Could you check a few things on this model? Use its own coordinates, in mm. A direction names the side the tool comes from. Round coordinates to 2 decimals unless told otherwise and drop trailing zeros. One line per item, written item: value. Start each with the question number.
(1) Thinking about a two-plate mould opening in Z: for faces 3 (the face through (2.849, -18.246, -5.028)), 4 (the face through (-9, -33.139, 3)), 5 (the face through (-2.9, -18.2, -5)), which applies, released by +Z, released by -Z, zero draft, split by the parting line, or undercut?
(2) Which directions (+Z, -Z, +X, -X, +Y, -Y) give clear straight access to the entire face, cutting with the end or side of a thin tool? Please do faces 1 (the face through (1.699, -3.219, -3.267)), 2 (the face through (-2.849, -18.246, 5.028)).
(3) If I drill on L1, parallel to X at y = -30.55, z = 0; L2, parallel to X at y = -12, z = 0; L3, parallel to Z at x = 0, y = -4.25, over which ranges is the centre line in solid material (lowest first)?
(4) I'm going to push flat-ended pins straight in: pin 1 Ø2 at (x, y) = (-2, -8.5) entering from -Z; pin 2 Ø4 at (y, z) = (-24.5, -1.5) entering from -X; pin 3 Ø1 at (x, z) = (-3, -5) entering from -Y; pin 4 Ø1.7 at (x, z) = (2.5, -5.5) entering from -Y. Where does each tip first touch, or does it pass through?
```python
from build123d import *

# Parameters (mm, degrees)
F0_R     = 9.525
F1_DEPTH = 15.24
F3_DEPTH = 8.89
F4_R     = 3.683
F5_DEPTH = 6.351
F8_R     = 2.54
F9_DEPTH = 15.24


# Not quite as in the source:
# - a feature names something its author has since deleted; it is built from what else it names


with BuildPart() as f1:
    # F0 (on Front) → F1 (new body)
    with BuildSketch(Plane.XZ):
        Circle(F0_R)
    extrude(amount=F1_DEPTH)

    # F2 (on face) → F3 (cut)
    with BuildSketch(Plane.XZ.offset(15.24)):
        Polygon((5.7785, -3.3362185305), (5.7785, 3.3362185305), (0, 6.672437061), (-5.7785, 3.3362185305), (-5.7785, -3.3362185305), (0, -6.672437061), align=None)
    extrude(amount=-F3_DEPTH, mode=Mode.SUBTRACT)

    # F4 (on face) → F5 (cut, through all)
    with BuildSketch(Plane.XZ.offset(6.35)):
        Circle(F4_R)
    extrude(amount=-F5_DEPTH, mode=Mode.SUBTRACT)

    # F6 (on Right) → F7 (revolve)
    with BuildSketch(Plane.YZ):
        with BuildLine():
            Line((-33.139064908, -6.672437061), (-33.139064908, -14.292437061))
            add(Edge.make_bspline(
                [(0, -9.4667123631), (-6.0169453004, -12.6291806394), (-11.4998287108, -14.4075187704), (-18.7425000775, -24.446910043), (-30.9530390066, -25.1909209173), (-33.139064908, -14.292437061)],
                knots=[0, 0, 0, 0, 0.3337672016, 0.635034675, 1, 1, 1, 1], degree=3))
            Line((0, -9.4667123631), (0, -6.672437061))
            Line((0, -6.672437061), (-33.139064908, -6.672437061))
        make_face()
    revolve(axis=Axis((0, -11.1619029194, 0), (0, -1, 0)))

    # F8
    f8_edges = [f1.edges().sort_by_distance(p)[0] for p in [
        (0, -33.139065, 6.672437),
    ]]
    fillet(f8_edges, radius=F8_R)

    # F9 (add): faces of the model
    f9_faces = [f1.faces().sort_by_distance(p)[0] for p in [
        (-3.069105432, -15.24, 5.315846542),
        (-6.138210864, -15.24, 0),
        (-3.069105432, -15.24, -5.315846542),
        (6.138210864, -15.24, 0),
        (3.069105432, -15.24, -5.315846542),
        (3.069105432, -15.24, 5.315846542),
    ]]
    extrude(f9_faces, amount=F9_DEPTH)


solid = f1.part
```
Found:
1. face 3: undercut
1. face 4: zero draft
1. face 5: undercut
2. face 1: +Y, -Y
2. face 2: -Y
3. L1: x = -20.79 to -6.67, 6.67 to 20.79
3. L2: x = -16.17 to -5.78, 5.78 to 16.17
3. L3: z = -11.61 to -3.68, 3.68 to 11.61
4. pin 1: stops at z = -14.19
4. pin 2: stops at x = -23.84
4. pin 3: stops at y = -30.48
4. pin 4: stops at y = -31.63
